```python
from build123d import *

# Parameters (mm, degrees)
SKETCH1_W           = 50.8
SKETCH1_H           = 25.4
BOSS_EXTRUDE1_DEPTH = 5.08
SKETCH2_R           = 6.35
BOSS_EXTRUDE5_DEPTH = 6.35
LPATTERN2_COUNT     = 4
LPATTERN2_PITCH     = 12.7
SKETCH7_W           = 6.35
SKETCH7_H           = 5.08
CUT_EXTRUDE2_DEPTH  = 5.08
CUT_EXTRUDE3_DEPTH  = 3.81
FILLET1_R           = 2.54
SKETCH2_5_R         = 2.416788658
CUT_EXTRUDE6_DEPTH  = 76.2


with BuildPart() as part:
    # Sketch1 → Boss-Extrude1 (new body)
    with BuildSketch(Plane.XY):
        Rectangle(SKETCH1_W, SKETCH1_H)
    extrude(amount=BOSS_EXTRUDE1_DEPTH)

    # Sketch2 → Boss-Extrude5 (add)
    with BuildSketch(Plane(origin=(25.4, 0, 0), x_dir=(0, 0, -1), z_dir=(1, 0, 0))):
        with Locations((0.853861474, 14.960926359)):
            Circle(SKETCH2_R)
    boss_extrude5 = extrude(amount=-BOSS_EXTRUDE5_DEPTH)

    # LPattern2: Boss-Extrude5 ×4
    with Locations(*[(-i * LPATTERN2_PITCH, 0, 0) for i in range(1, LPATTERN2_COUNT)]):
        add(boss_extrude5)

    # Sketch7 → Cut-Extrude2 (cut)
    with BuildSketch(Plane(origin=(0, 12.7, 0), x_dir=(1, 0, 0), z_dir=(0, 1, 0))):
        with Locations((15.875, -2.54)):
            Rectangle(SKETCH7_W, SKETCH7_H)
        with Locations((3.175, -2.54)):
            Rectangle(SKETCH7_W, SKETCH7_H)
        with Locations((-9.525, -2.54)):
            Rectangle(SKETCH7_W, SKETCH7_H)
        with Locations((-22.225, -2.54)):
            Rectangle(SKETCH7_W, SKETCH7_H)
    extrude(amount=-CUT_EXTRUDE2_DEPTH, mode=Mode.SUBTRACT)

    # Sketch8 → Cut-Extrude3 (cut)
    with BuildSketch(Plane(origin=(0, 0, 0), x_dir=(-1, 0, 0), z_dir=(0, 0, -1))):
        Polygon((-19.05, 7.62), (-19.05, 8.668596061), (-25.4, 8.668596061), (-25.4, -12.7), (25.4, -12.7), (25.4, 7.62), (19.05, 7.62), (19.05, 8.668596061), (12.7, 8.668596061), (12.7, 7.62), (6.35, 7.62), (6.35, 8.668596061), (0, 8.668596061), (0, 7.62), (-6.35, 7.62), (-6.35, 8.668596061), (-12.7, 8.668596061), (-12.7, 7.62), align=None)
    extrude(amount=-CUT_EXTRUDE3_DEPTH, mode=Mode.SUBTRACT)

    # Fillet1
    fillet1_edges = [part.edges().sort_by_distance(p)[0] for p in [
        (25.4, -12.7, 4.445),
        (-25.4, -12.7, 4.445),
    ]]
    fillet(fillet1_edges, radius=FILLET1_R)

    # Sketch2<5> → Cut-Extrude6 (cut)
    with BuildSketch(Plane(origin=(25.4, 0, 0), x_dir=(0, 0, -1), z_dir=(1, 0, 0))):
        with Locations((0.853861474, 14.960926359)):
            Circle(SKETCH2_5_R)
    extrude(amount=-CUT_EXTRUDE6_DEPTH, mode=Mode.SUBTRACT)


solid = part.part
```
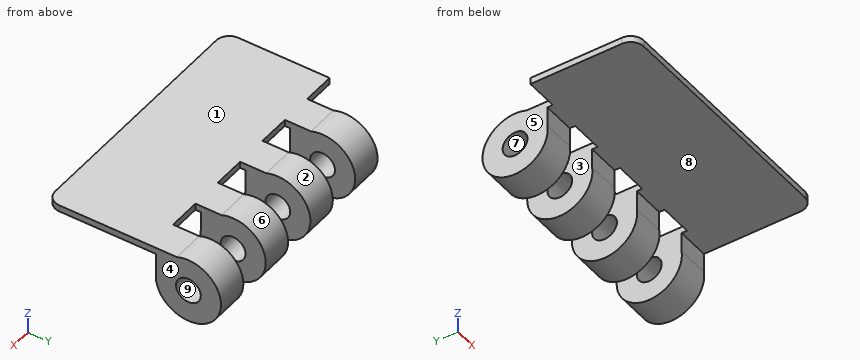
Design review of the part built by this model. Coordinates are the model's own, in mm. Face numbers are marked on the shaded views. A direction names the side the tool comes from. Round coordinates to 2 decimals unless told otherwise and drop trailing zeros. Write each loop counter-clockwise with the first axis right and the second up, starting at its lowest first coordinate (ties: lowest second). Pieces come first, ordered by that corner, then holes.
Item 1: We need section A-A on z = -5. Write out the cut boundary in (x, y).
Item 2: The part is to be moulded in two halves that separate along Y. For the marked faces 6, 7, 8 and 9, say which applies: +Y half, -Y half, draft (parallel to the pull), parting line (faces both ways), or undercut.
Item 3: Clearance check with flat-ended pins moving along their axes: pin 1 Ø2 at (x, y) = (-1.5, 11) entering from -Z; pin 2 Ø10.5 at (x, y) = (11.5, -3.5) entering from -Z; pin 3 Ø1.9 at (x, z) = (10.5, 2.5) entering from -Y; pin 4 Ø4 at (x, z) = (-2, 2.5) entering from -Y. State where each tip first meets the part, or that it passes through.
Item 4: We need section C-C on x = 17.5. Write out the cut boundary in (y, z).
Item 5: For the marked faces 1, 2, 3, 4 and 5, list the 3-axis set-ups (+Z, -Z, +X, -X, +Y, -Y) from which the entire face can be reached by the end or side of a thin tool; tool diameter is ignored.
Item 6: We need section B-B on y = 12. Write out the cut boundary in (x, z), and give its area (3 significant figures).
Item 7: We need section D-D on z = -1.25. State how many separate pieces and enclosed holes the cut face has, and give its area (3 significant figures).
Item 8: For probe 1 along X at (y, z) = (13, 4.75); probe 2 along Z at (x, y) = (11, 4.5), list the stretches that pass through material, from the lowest coordinate up.
Returned:
1. outline: (-19.05, 10.15) - (-12.7, 10.15) - (-12.7, 19.77) - (-19.05, 19.77) - close; (-6.35, 10.15) - (0, 10.15) - (0, 19.77) - (-6.35, 19.77) - close; (6.35, 10.15) - (12.7, 10.15) - (12.7, 19.77) - (6.35, 19.77) - close; (19.05, 10.15) - (25.4, 10.15) - (25.4, 19.77) - (19.05, 19.77) - close
2. face 6: parting line
2. face 7: undercut
2. face 8: draft
2. face 9: undercut
3. pin 1: stops at z = -6.47
3. pin 2: stops at z = 3.81
3. pin 3: stops at y = 8.67
3. pin 4: stops at y = -12.7
4. outline: (-12.7, 3.81) - (7.62, 3.81) - (7.62, 5.08) - (-12.7, 5.08) - close
5. face 1: +Z, +X, -X, -Y
5. face 2: +X, -X
5. face 3: +Z, -Z, +Y
5. face 4: +Z, -Z, +X, +Y, -Y
5. face 5: +Z, -Z, -X, +Y
6. outline: (-19.05, -6.47) - (-12.7, -6.47) - (-12.7, 5.08) - (-19.05, 5.08) - close; (-6.35, -6.47) - (0, -6.47) - (0, 5.08) - (-6.35, 5.08) - close; (6.35, -6.47) - (12.7, -6.47) - (12.7, 5.08) - (6.35, 5.08) - close; (19.05, -6.47) - (25.4, -6.47) - (25.4, 5.08) - (19.05, 5.08) - close
6. area: 293 mm2
7. separate pieces: 8
7. enclosed holes: 0
7. area: 201 mm2
8. probe 1: x = -19.05 to -12.7, -6.35 to 0, 6.35 to 12.7, 19.05 to 25.4
8. probe 2: z = 3.81 to 5.08
